Design review of the part built by this model. Coordinates are the model's own, in mm. Face numbers are marked on the shaded views. A direction names the side the tool comes from. Coordinates: 2 decimals unless noted, no trailing zeros. Write each loop counter-clockwise with the first axis right and the second up, starting at its lowest first coordinate (ties: lowest second). Pieces come first, ordered by that corner, then holes.
Q1. For the marked faces 5, 6, 7, 8 and 9, list the 3-axis set-ups (+Z, -Z, +X, -X, +Y, -Y) from which the entire face can be reached by the end or side of a thin tool; tool diameter is ignored.
Q2. Take a section at C-C, the plane x = 4. Write out the cut boundary in (y, z).
Q3. Take a section at B-B, the plane x = 7. Write out the cut boundary in (y, z).
Q4. For pin 1 Ø1.2 at (x, z) = (7, 0) entering from +Y; pin 2 Ø0.8 at (y, z) = (-2.5, 0.5) entering from +X; pin 3 Ø2 at (x, z) = (-7.5, -1) entering from -Y; pin 4 Ø1.2 at (y, z) = (1.5, -1) entering from -X, all flat-tipped, find the tip position at first contact; note any pin that passes through.
Q5. For L1, parallel to Z at x = 7, y = 4.6; L2, parallel to Y at x = 8, z = -0.55; L3, parallel to Y at x = 1.75, z = 0.85, list the stretches that pass through material, from the lowest coordinate up.
Q6. Take a section at D-D, the plane z = 1.6. Write out the cut boundary in (x, y).
Q7. Take a section at A-A, the plane y = -1. Write out the cut boundary in (x, z), plus the area to 3 significant figures.
Q8. The part is to be moulded in two halves that separate along X. For the marked faces 1, 2, 3 and 4, say which applies: released by +X, released by -X, zero draft, split by the parting line, or undercut.
from build123d import *

# Parameters (mm, degrees)
SKETCH2_W                  = 10
SKETCH2_H                  = 4
BOSS_EXTRUDE1_DEPTH        = 5
SKETCH3_W                  = 6
SKETCH3_H                  = 2
CUT_EXTRUDE1_DEPTH         = 0.5
SKETCH4_W                  = 4
SKETCH4_H                  = 0.5
BOSS_EXTRUDE2_DEPTH        = 4
SKETCH5_R                  = 1
CUT_EXTRUDE2_DEPTH         = 1.5
FILLET1_R                  = 1
SKETCH6_W                  = 2.5
SKETCH6_H                  = 2
BOSS_EXTRUDE3_DEPTH        = 3.5
FILLET2_R                  = 0.8
SKETCH7_W                  = 0.1
SKETCH7_H                  = 2
BOSS_EXTRUDE4_DEPTH        = 0.1
SKETCH8_W                  = 9.7
SKETCH8_H                  = 3.7
CUT_EXTRUDE3_DEPTH         = 0.1
SKETCH9_W                  = 0.1
SKETCH9_H                  = 2.5
BOSS_EXTRUDE5_DEPTH        = 4
FILLET3_R                  = 1
SKETCH10_R                 = 0.5
CUT_EXTRUDE4_DEPTH         = 10.05
LPATTERN1_COUNT            = 2
LPATTERN1_PITCH            = 2.5
FILLET3_OF_LPATTERN1_R     = 1
LPATTERN1_COL_COUNT        = 2
LPATTERN1_COL_PITCH        = 2.5
FILLET3_OF_LPATTERN1_COL_R = 1


with BuildPart() as part:
    # Sketch2 → Boss-Extrude1 (new body)
    with BuildSketch(Plane(origin=(0, 0, 0), x_dir=(1, 0, 0), z_dir=(0, 1, 0))):
        Rectangle(SKETCH2_W, SKETCH2_H)
    extrude(amount=BOSS_EXTRUDE1_DEPTH)

    # Sketch3 → Cut-Extrude1 (cut)
    with BuildSketch(Plane(origin=(0, 5, 0), x_dir=(1, 0, 0), z_dir=(0, 1, 0))):
        Rectangle(SKETCH3_W, SKETCH3_H)
    extrude(amount=-CUT_EXTRUDE1_DEPTH, mode=Mode.SUBTRACT)

    # Sketch4 → Boss-Extrude2 (add)
    with BuildSketch(Plane(origin=(5, 0, 0), x_dir=(0, 0, -1), z_dir=(1, 0, 0))):
        with Locations((0, 4.75)):
            Rectangle(SKETCH4_W, SKETCH4_H)
    boss_extrude2 = extrude(amount=BOSS_EXTRUDE2_DEPTH)

    # Sketch5 → Cut-Extrude2 (cut, through all)
    with BuildSketch(Plane.XZ.offset(-4.5)):
        with Locations((7, 0)):
            Circle(SKETCH5_R)
    cut_extrude2 = extrude(amount=-CUT_EXTRUDE2_DEPTH, mode=Mode.SUBTRACT)

    # Mirror3: Boss-Extrude2, Cut-Extrude2 across plane
    add(boss_extrude2.mirror(Plane(origin=(0, 0, 0), x_dir=(0, 0, 1), z_dir=(1, 0, 0))))
    add(cut_extrude2.mirror(Plane(origin=(0, 0, 0), x_dir=(0, 0, 1), z_dir=(1, 0, 0))), mode=Mode.SUBTRACT)

    # Fillet1
    fillet1_edges = [part.edges().sort_by_distance(p)[0] for p in [
        (9, 4.75, 2),
        (9, 4.75, -2),
        (-9, 4.75, 2),
        (-9, 4.75, -2),
    ]]
    fillet(fillet1_edges, radius=FILLET1_R)

    # Sketch6 → Boss-Extrude3 (add)
    with BuildSketch(Plane(origin=(0, 4.5, 0), x_dir=(1, 0, 0), z_dir=(0, 1, 0))):
        with Locations((-1.53254506, 0)):
            Rectangle(SKETCH6_W, SKETCH6_H)
    extrude(amount=BOSS_EXTRUDE3_DEPTH)

    # Fillet2
    fillet2_edges = [part.edges().sort_by_distance(p)[0] for p in [
        (-2.78254506, 8, 0),
        (-0.28254506, 8, 0),
    ]]
    fillet(fillet2_edges, radius=FILLET2_R)

    # Sketch7 → Boss-Extrude4 (add)
    with BuildSketch(Plane(origin=(0, 4.5, 0), x_dir=(1, 0, 0), z_dir=(0, 1, 0))):
        with Locations((-0.23254506, 0)):
            Rectangle(SKETCH7_W, SKETCH7_H)
        with Locations((-2.83254506, 0)):
            Rectangle(SKETCH7_W, SKETCH7_H)
    extrude(amount=BOSS_EXTRUDE4_DEPTH)

    # Sketch8 → Cut-Extrude3 (cut)
    with BuildSketch(Plane.XZ):
        Rectangle(SKETCH8_W, SKETCH8_H)
    extrude(amount=-CUT_EXTRUDE3_DEPTH, mode=Mode.SUBTRACT)

    # Sketch9 → Boss-Extrude5 (add)
    with BuildSketch(Plane.XZ.offset(-0.1)):
        Rectangle(SKETCH9_W, SKETCH9_H)
    boss_extrude5 = extrude(amount=BOSS_EXTRUDE5_DEPTH)

    # Fillet3
    fillet3_edges = [part.edges().sort_by_distance(p)[0] for p in [
        (0, -3.9, 1.25),
        (0, -3.9, -1.25),
    ]]
    fillet(fillet3_edges, radius=FILLET3_R)

    # Sketch10 → Cut-Extrude4 (cut, through all)
    with BuildSketch(Plane.ZY.offset(0.05)):
        with Locations((0, -2.4)):
            Circle(SKETCH10_R)
    cut_extrude4 = extrude(amount=-CUT_EXTRUDE4_DEPTH, mode=Mode.SUBTRACT)

    # LPattern1: Boss-Extrude5, Cut-Extrude4 ×2
    with Locations(*[(i * LPATTERN1_PITCH, 0, 0) for i in range(1, LPATTERN1_COUNT)]):
        add(boss_extrude5)
        add(cut_extrude4, mode=Mode.SUBTRACT)

    # Fillet3 of LPattern1
    fillet3_of_lpattern1_edges = [part.edges().sort_by_distance(p)[0] for p in [
        (2.5, -3.9, 1.25),
        (2.5, -3.9, -1.25),
    ]]
    fillet(fillet3_of_lpattern1_edges, radius=FILLET3_OF_LPATTERN1_R)

    # LPattern1 col: Boss-Extrude5, Cut-Extrude4 ×2
    with Locations(*[(-i * LPATTERN1_COL_PITCH, 0, 0) for i in range(1, LPATTERN1_COL_COUNT)]):
        add(boss_extrude5)
        add(cut_extrude4, mode=Mode.SUBTRACT)

    # Fillet3 of LPattern1 col
    fillet3_of_lpattern1_col_edges = [part.edges().sort_by_distance(p)[0] for p in [
        (-2.5, -3.9, 1.25),
        (-2.5, -3.9, -1.25),
    ]]
    fillet(fillet3_of_lpattern1_col_edges, radius=FILLET3_OF_LPATTERN1_COL_R)


solid = part.part
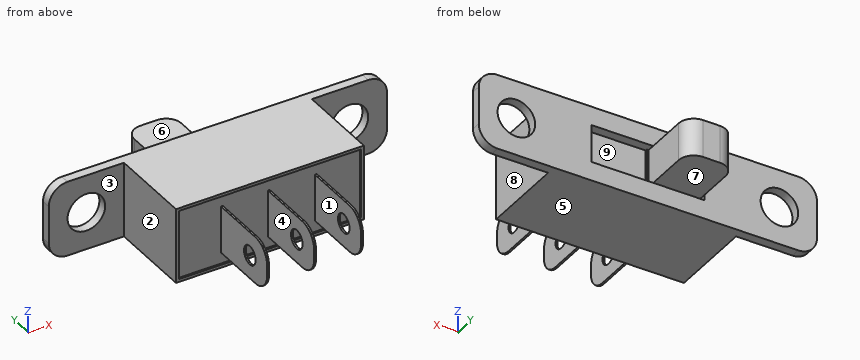
Responses:
1. face 5: -Z, +X, -X, +Y, -Y
1. face 6: +Z, +X, -X, +Y
1. face 7: -Z, +X, -X, +Y
1. face 8: +Z, -Z, +X, -Y
1. face 9: +Y
2. outline: (0, -2) - (5, -2) - (5, 2) - (0, 2) - (0, 1.85) - (0.1, 1.85) - (0.1, -1.85) - (0, -1.85) - close
3. outline: (4.5, -2) - (5, -2) - (5, -1) - (4.5, -1) - close; (4.5, 1) - (5, 1) - (5, 2) - (4.5, 2) - close
4. pin 1: passes through
4. pin 2: stops at x = 2.55
4. pin 3: stops at y = 4.5
4. pin 4: stops at x = -5
5. L1: z = -2 to -1, 1 to 2
5. L2: y = 4.5 to 5
5. L3: y = 0.1 to 4.5
6. outline: (-8.8, 4.5) - (-5, 4.5) - (-5, 0) - (-4.85, 0) - (-4.85, 0.1) - (4.85, 0.1) - (4.85, 0) - (5, 0) - (5, 4.5) - (8.8, 4.5) - (8.8, 5) - (-8.8, 5) - close
7. outline: (-2.55, -1.25) - (-2.45, -1.25) - (-2.45, 1.25) - (-2.55, 1.25) - close; (-0.05, -1.25) - (0.05, -1.25) - (0.05, 1.25) - (-0.05, 1.25) - close; (2.45, -1.25) - (2.55, -1.25) - (2.55, 1.25) - (2.45, 1.25) - close
7. area: 0.750 mm2
8. face 1: undercut
8. face 2: released by -X
8. face 3: zero draft
8. face 4: undercut
